from build123d import *

# Parameters (mm, degrees)
SKETCH1_W               = 25.4
SKETCH1_H               = 9.525
SKETCH1_R               = 3.175
BOSS_EXTRUDE1_DEPTH     = 3.175
CUT_EXTRUDE1_DEPTH      = 14.930255965
CUT_EXTRUDE1_DEPTH_BACK = 14.930255965
SKETCH2_R               = 2.4892


with BuildPart() as part:
    # Sketch1 → Boss-Extrude1 (new, symmetric)
    with BuildSketch(Plane.XY):
        Rectangle(SKETCH1_W, SKETCH1_H)
        Circle(SKETCH1_R, mode=Mode.SUBTRACT)
    extrude(amount=BOSS_EXTRUDE1_DEPTH, both=True)

    # Sketch2 → Cut-Extrude1 (cut, two sides: drawn at the far end of the back side and taken through both)
    with BuildSketch(Plane(origin=(0, 0, 0), x_dir=(1, 0, 0), z_dir=(0, 1, 0)).offset(-CUT_EXTRUDE1_DEPTH_BACK)):
        with Locations(Location((6.35, 0, 0), (0, 0, 270))):
            Circle(SKETCH2_R)
        with Locations(Location((-6.35, 0, 0), (0, 0, 270))):
            Circle(SKETCH2_R)
    extrude(amount=CUT_EXTRUDE1_DEPTH + CUT_EXTRUDE1_DEPTH_BACK, mode=Mode.SUBTRACT)


solid = part.part
Work out the finished part from the listing and answer in its coordinate system (mm). Coordinates: 2 decimals unless noted, no trailing zeros. Order: outer loops, then holes, each group sorted by start corner. A loop starts at its lowest first (then second) coordinate and runs counter-clockwise, first axis right, second up. Notation, with made-up numbers: (-38, 85.5) - (-11, 85.5) arc R29 cw to (-11, 123.5) - close; hole circle Ø10 at (87, 55.5). An arc over 180 degrees is marked (long way). Put each result on its own line as item: value. Start each with the question number.
1) Find section B-B (z = 0). State how many separate pieces and enclosed holes the cut face has, plus the area to 3 significant figures.
2) Find section C-C (x = 0). Give the vertices of the cut face in (y, z) (1 decimal).
3) For a pull along Z with two mould halves and no side action, classify faces 1 (the flat face through (-12.7, 0, 0)), 2 (the cylindrical face through (-4.25, -0.07, 1.34)), 3 (the flat face through (-3, 2, -3.175)) as released by +Z, released by -Z, zero draft, split by the parting line, or undercut.
4) Find the intervals of material crossed by line 1 (Z direction, x = 6.35, y = -1) (3 decimals); line 2 (X direction, y = 2.25, z = -1); line 3 (X direction, y = 2.5, z = 0), in increasing order. Write a range as from..to.
5) Find section A-A (y = 0). Give the vertices of the cut face in (x, z) (3 decimals), plus the area to 3 significant figures.
Results list:
1. separate pieces: 3
1. enclosed holes: 1
1. area: 115 mm^2
2. outline: (-4.8, -3.2) - (-3.2, -3.2) - (-3.2, 3.2) - (-4.8, 3.2) - close; (3.2, -3.2) - (4.8, -3.2) - (4.8, 3.2) - (3.2, 3.2) - close
3. face 1: zero draft
3. face 2: undercut
3. face 3: released by -Z
4. line 1: z = -3.175..-2.489, 2.489..3.175
4. line 2: x = -12.7..-8.63, -4.07..-2.24, 2.24..4.07, 8.63..12.7
4. line 3: x = -12.7..-8.84, -3.86..-1.96, 1.96..3.86, 8.84..12.7
5. outline: (-12.7, -3.175) - (-3.175, -3.175) - (-3.175, 3.175) - (-12.7, 3.175) - close; (3.175, -3.175) - (12.7, -3.175) - (12.7, 3.175) - (3.175, 3.175) - close; hole circle Ø4.978 at (-6.35, 0); hole circle Ø4.978 at (6.35, 0)
5. area: 82.0 mm^2
